The listing builds one solid part. Answer for the finished solid, in the listing's coordinates (mm). A direction names the side the tool comes from. Round coordinates to 2 decimals unless told otherwise and drop trailing zeros. Write each loop counter-clockwise with the first axis right and the second up, starting at its lowest first coordinate (ties: lowest second). Pieces come first, ordered by that corner, then holes.
from build123d import *

# Parameters (mm, degrees)
SKETCH1_R           = 12.2
BOSS_EXTRUDE1_DEPTH = 31
SKETCH2_R           = 12.5
BOSS_EXTRUDE2_DEPTH = 21
SKETCH3_R           = 3.5
BOSS_EXTRUDE3_DEPTH = 2.5
SKETCH4_R           = 2
BOSS_EXTRUDE4_DEPTH = 8
SKETCH5_R           = 7
BOSS_EXTRUDE5_DEPTH = 9
SKETCH6_W           = 12
SKETCH6_H           = 7
BOSS_EXTRUDE6_DEPTH = 4
SKETCH7_R           = 1.5
CUT_EXTRUDE1_DEPTH  = 7


with BuildPart() as part:
    # Sketch1 → Boss-Extrude1 (new body)
    with BuildSketch(Plane.XY):
        Circle(SKETCH1_R)
    extrude(amount=BOSS_EXTRUDE1_DEPTH)

    # Sketch2 → Boss-Extrude2 (add)
    with BuildSketch(Plane.XY.offset(31)):
        with Locations(Location((0, 0, 0), (0, 0, 180))):
            Circle(SKETCH2_R)
    extrude(amount=BOSS_EXTRUDE2_DEPTH)

    # Sketch3 → Boss-Extrude3 (add)
    with BuildSketch(Plane.XY.offset(52)):
        Circle(SKETCH3_R)
    extrude(amount=BOSS_EXTRUDE3_DEPTH)

    # Sketch4 → Boss-Extrude4 (add)
    with BuildSketch(Plane.XY.offset(54.5)):
        Circle(SKETCH4_R)
    extrude(amount=BOSS_EXTRUDE4_DEPTH)

    # Sketch5 → Boss-Extrude5 (add)
    with BuildSketch(Plane(origin=(0, 0, 0), x_dir=(-1, 0, 0), z_dir=(0, 0, -1))):
        Circle(SKETCH5_R)
    extrude(amount=BOSS_EXTRUDE5_DEPTH)

    # Sketch6 → Boss-Extrude6 (add)
    with BuildSketch(Plane(origin=(0, 0, 0), x_dir=(-1, 0, 0), z_dir=(0, 0, -1))):
        with Locations((0, -11)):
            Rectangle(SKETCH6_W, SKETCH6_H)
    extrude(amount=BOSS_EXTRUDE6_DEPTH)

    # Sketch7 → Cut-Extrude1 (cut)
    with BuildSketch(Plane.XY.offset(52)):
        with Locations((-9, 0)):
            Circle(SKETCH7_R)
        with Locations((9, 0)):
            Circle(SKETCH7_R)
    extrude(amount=-CUT_EXTRUDE1_DEPTH, mode=Mode.SUBTRACT)


solid = part.part
1. Given pin 1 (3.5 mm diameter, centred on x = -8.5, y = -0.5, fed in from +Z); pin 2 (3 mm diameter, centred on x = 1, z = -2, fed in from +Y); pin 3 (12 mm diameter, centred on x = 0, z = 31.5, fed in from -Y), each flat-ended and moving along its own axis, determine where each tip first touches the part or whether it passes through.
Geometry says:
pin 1: stops at z = 52
pin 2: stops at y = 7
pin 3: stops at y = -12.5
2. A tool of negligible diameter and unlimited length cuts with its end or side. For faces 1 (the face through (-6, -11, -2)), 2 (the face through (6, -11, -2)), 3 (the face through (-10.5, 0.07, 48.55)), 4 (the face through (-12.19, 0.54, 15.28)), from which of +Z, -Z, +X, -X, +Y, -Y can it reach the whole face along a straight path? Write none if from no direction.
Geometry says:
face 1: -Z, -X, -Y
face 2: -Z, +X, -Y
face 3: +Z
face 4: none
3. Section B-B on y = 0 is taken. Determine the outline of the cut face in (x, z).
Geometry says:
outline: (-12.5, 31) - (-12.2, 31) - (-12.2, 0) - (-7, 0) - (-7, -9) - (7, -9) - (7, 0) - (12.2, 0) - (12.2, 31) - (12.5, 31) - (12.5, 52) - (10.5, 52) - (10.5, 45) - (7.5, 45) - (7.5, 52) - (3.5, 52) - (3.5, 54.5) - (2, 54.5) - (2, 62.5) - (-2, 62.5) - (-2, 54.5) - (-3.5, 54.5) - (-3.5, 52) - (-7.5, 52) - (-7.5, 45) - (-10.5, 45) - (-10.5, 52) - (-12.5, 52) - close
4. Straight lines are drawn through the part: line 1 along Y through (x, z) = (-0.25, 22); line 2 along Z through (x, y) = (4.5, -1); line 3 along Z through (x, y) = (7.5, 3.75). For each, find the intervals that lie inside material, in ascending order.
Geometry says:
line 1: y = -12.2 to 12.2
line 2: z = -9 to 52
line 3: z = 0 to 52
5. Section C-C on z = 56.5 is taken. Determine the outline of the cut face in (x, y).
Geometry says:
outline: circle Ø4 at (0, 0)
6. For a pull along Y with two mould halves and no side action, classify faces 5 (the face through (0, -14.5, -2)), 6 (the face through (9, 0, 45)), 7 (the face through (2, -2, 54.5)) as released by +Y, released by -Y, zero draft, split by the parting line, or undercut.
Geometry says:
face 5: released by -Y
face 6: undercut
face 7: zero draft
7. Section D-D on y = 8.5 is taken. Determine the outline of the cut face in (x, z).
Geometry says:
outline: (-9.17, 31) - (-8.75, 31) - (-8.75, 0) - (8.75, 0) - (8.75, 31) - (9.17, 31) - (9.17, 52) - (-9.17, 52) - close
8. Section A-A on x = 0 is taken. Determine the outline of the cut face in (y, z).
Geometry says:
outline: (-14.5, -4) - (-7.5, -4) - (-7.5, 0) - (-7, 0) - (-7, -9) - (7, -9) - (7, 0) - (12.2, 0) - (12.2, 31) - (12.5, 31) - (12.5, 52) - (3.5, 52) - (3.5, 54.5) - (2, 54.5) - (2, 62.5) - (-2, 62.5) - (-2, 54.5) - (-3.5, 54.5) - (-3.5, 52) - (-12.5, 52) - (-12.5, 31) - (-12.2, 31) - (-12.2, 0) - (-14.5, 0) - close
